Design review of the part built by this model. Coordinates are the model's own, in mm. Face numbers are marked on the shaded views. A direction names the side the tool comes from. Give positions to 0.01 mm unless a question says otherwise; leave off trailing zeros. Order: outer loops, then holes, each group sorted by start corner. A loop starts at its lowest first (then second) coordinate and runs counter-clockwise, first axis right, second up. Notation, with made-up numbers: (57, 13.25) -> (80, 13.25) arc R15 ccw to (80, 24.25) -> close; hole circle Ø5 at (22.25, 2). An arc over 180 degrees is marked (long way). One line per item, written item: value. Start each with the question number.
1) Wall thickness on line 1 along X through (y, z) = (1.55, 0); line 2 along Y through (x, z) = (-0.25, 5.25); line 3 along X through (y, z) = (0.4, 1.25) (3 decimals): over which ranges is each line inside the solid? List them lowest first. Write a range as from..to.
2) Consider section C-C (y = -0.65). State the section outline as (x, z) points.
3) Tool access review of the marked faces 4 and 5: name each direction out of +Z, -Z, +X, -X, +Y, -Y from which nothing blocks a thin tool from reaching the whole face with its end or side.
4) Consider section D-D (z = 3.75). State the section outline as (x, y) points (1 decimal).
5) For pin 1 (6 mm diameter, centred on x = 0, z = 0, fed in from +Y); pin 2 (2 mm diameter, centred on y = 2.5, z = -4.5, fed in from +X); pin 3 (1 mm diameter, centred on y = -1, z = 2, fed in from +X), all flat-tipped, find the tip position at first contact; note any pin that passes through.
6) The part is to be moulded in two halves that separate along Z. For the marked faces 1, 2 and 3, say which applies: released by +Z, released by -Z, zero draft, split by the parting line, or undercut.
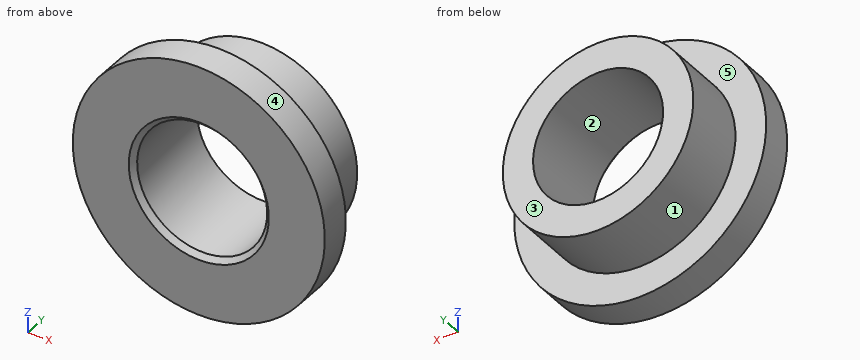
from build123d import *

# Parameters (mm, degrees)
SKETCH2_R           = 4.8006
BOSS_EXTRUDE1_DEPTH = 3.175
SKETCH3_R           = 6.35
BOSS_EXTRUDE2_DEPTH = 1.5875
SKETCH4_R           = 3.2766
CUT_EXTRUDE1_DEPTH  = 11.164959727
CHAMFER1_SIZE       = 0.254


with BuildPart() as part:
    # Sketch2 → Boss-Extrude1 (new body)
    with BuildSketch(Plane(origin=(0, 0, 0), x_dir=(1, 0, 0), z_dir=(0, 1, 0))):
        with Locations(Location((0, 0, 0), (0, 0, 270))):
            Circle(SKETCH2_R)
    extrude(amount=BOSS_EXTRUDE1_DEPTH)

    # Sketch3 → Boss-Extrude2 (add)
    with BuildSketch(Plane(origin=(0, 0, 0), x_dir=(-1, 0, 0), z_dir=(0, -1, 0))):
        with Locations(Location((0, 0, 0), (0, 0, 90))):
            Circle(SKETCH3_R)
    extrude(amount=BOSS_EXTRUDE2_DEPTH)

    # Sketch4 → Cut-Extrude1 (cut, through all)
    with BuildSketch(Plane(origin=(0, 3.175, 0), x_dir=(1, 0, 0), z_dir=(0, 1, 0))):
        with Locations(Location((0, 0, 0), (0, 0, 270))):
            Circle(SKETCH4_R)
    extrude(amount=-CUT_EXTRUDE1_DEPTH, mode=Mode.SUBTRACT)

    # Chamfer1
    chamfer1_edges = [part.edges().sort_by_distance(p)[0] for p in [
        (0, -1.5875, -3.2766),
    ]]
    chamfer(chamfer1_edges, length=CHAMFER1_SIZE)


solid = part.part
Checked values:
1. line 1: x = -4.8..-3.28, 3.28..4.8
1. line 2: y = -1.59..0
1. line 3: x = -4.635..-3.029, 3.029..4.635
2. outline: circle Ø12.7 at (0, 0); hole circle Ø6.55 at (0, 0)
3. face 4: +Y, -Y
3. face 5: +Y
4. outline: (-5.1, -1.6) -> (5.1, -1.6) -> (5.1, 0) -> (3, 0) -> (3, 3.2) -> (-3, 3.2) -> (-3, 0) -> (-5.1, 0) -> close
5. pin 1: passes through
5. pin 2: stops at x = 3.29
5. pin 3: stops at x = 6.17
6. face 1: split by the parting line
6. face 2: undercut
6. face 3: zero draft
